Study the drawing (mm; zero at the part's minimum x, y, z) and answer. Give positions to 0.01 mm unless a question says otherwise; leave off trailing zeros. Loops run counter-clockwise (first coordinate to the right, second up) from the corner with the lowest first, then second, coordinate; pieces in that order, holes last. Notation, with made-up numbers: (46.5, 12) -> (55.5, 12) arc R27 cw to (55.5, 36) -> close; hole circle Ø9 at (77.25, -19). An arc over 180 degrees is marked (long way). One line per question, with ' | ' between items. Start each with the question number.
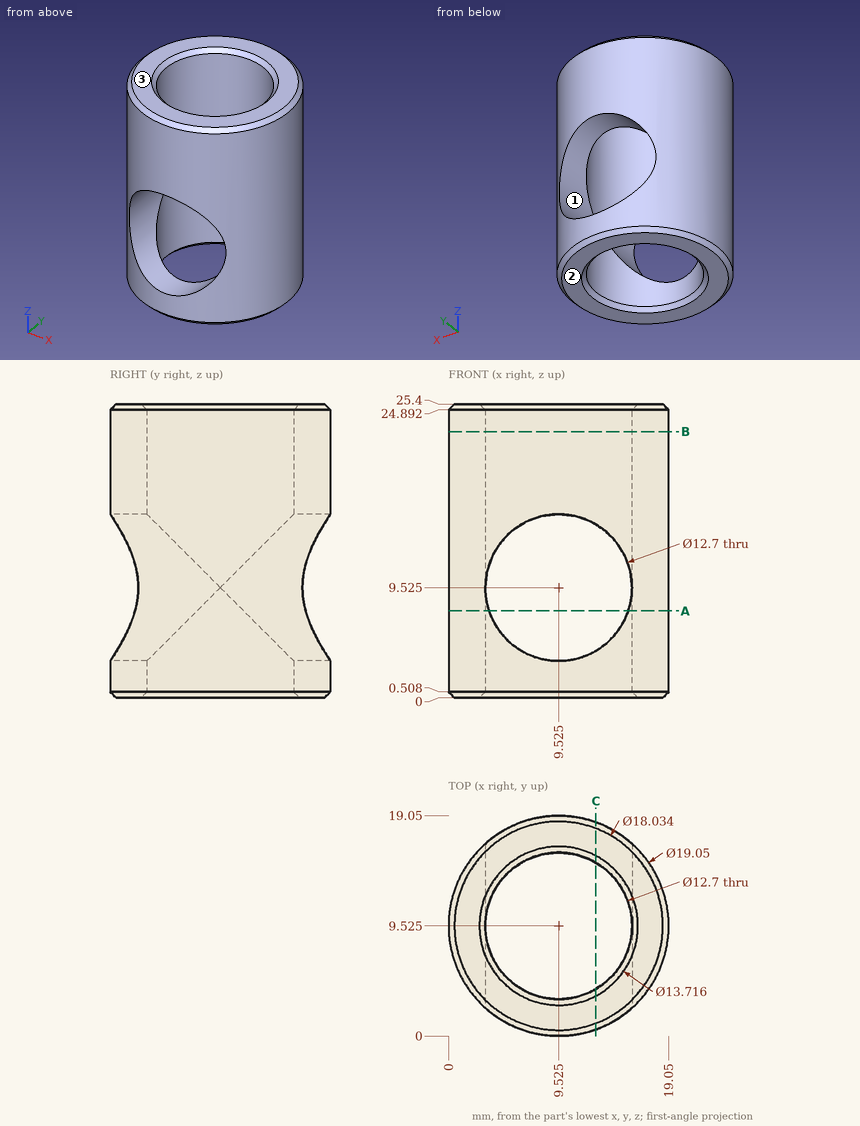
1. Straight lines are drawn through the part: L1, parallel to X at y = 9.5, z = 21.5; L2, parallel to Z at x = 9.25, y = 2.25; L3, parallel to X at y = 14.25, z = 3.75. For each, find the intervals that lie inside material, in ascending order.
2. Determine the mould class of the marked faces 1, 2 and 3 for opening direction Z: released by +Z, released by -Z, zero draft, split by the parting line, or undercut.
3. The part is cut by section C-C (x = 12.75). Count the separate pieces of the cut face and the enclosed holes in it, plus the area to 3 significant figures.
4. The part is cut by section A-A (z = 7.5). Write down the section's boundary in (x, y) (3 decimals).
5. Each of these flat-tipped pins is pushed along its axis until it touches: pin 1 Ø10 at (y, z) = (4, 21.5) entering from +X; pin 2 Ø5 at (x, z) = (13.5, 19.5) entering from -Y; pin 3 Ø6 at (x, z) = (9, 13.5) entering from -Y; pin 4 Ø7.5 at (x, z) = (9.525, 9.525) entering from +Y. Where does it stop, or does it pass through?
6. The part is cut by section B-B (z = 23). Write down the section's boundary in (x, y) (3 decimals), plus the area to 3 significant figures.
Check sheet entries:
1) L1: x = 0 to 3.18, 15.87 to 19.05 | L2: z = 0 to 3.18, 15.87 to 25.4 | L3: x = 1.25 to 5.28, 13.77 to 17.8
2) face 1: undercut | face 2: released by -Z | face 3: released by +Z
3) separate pieces: 4 | enclosed holes: 0 | area: 99.9 mm^2
4) outline: (3.507, 2.142) -> (3.507, 7.5) arc R6.35 cw to (3.507, 11.55) -> (3.507, 16.908) arc R9.525 ccw to start; (15.543, 2.142) arc R9.525 ccw to (15.543, 16.908) -> (15.543, 11.55) arc R6.35 cw to (15.543, 7.5) -> close
5) pin 1: stops at x = 19.04 | pin 2: stops at y = 0.11 | pin 3: stops at y = 0 | pin 4: passes through
6) outline: circle Ø19.05 at (9.525, 9.525); hole circle Ø12.7 at (9.525, 9.525) | area: 158 mm^2
